from build123d import *

# Parameters (mm, degrees)
F0_R     = 63.5
F1_DEPTH = 7.62
F2_R     = 12.7
F3_DEPTH = 7.621


with BuildPart() as f1:
    # F0 (on Front) → F1 (new body)
    with BuildSketch(Plane.XZ):
        Circle(F0_R)
    extrude(amount=F1_DEPTH)

    # F2 (on Front) → F3 (cut, through all)
    with BuildSketch(Plane.XZ):
        with Locations((-28.595986, 36.92016)):
            Circle(F2_R)
        with Locations((-43.949804, -15.787442)):
            Circle(F2_R)
        with Locations((1.433513, -46.677336)):
            Circle(F2_R)
        with Locations((44.835764, -13.060738)):
            Circle(F2_R)
        with Locations((26.276513, 38.605356)):
            Circle(F2_R)
    extrude(amount=F3_DEPTH, mode=Mode.SUBTRACT)


solid = f1.part
Input: part model. Units: mm. Frame: model coordinates. Coordinates: 2 decimals unless noted, no trailing zeros. Loops run counter-clockwise (first coordinate to the right, second up) from the corner with the lowest first, then second, coordinate; pieces in that order, holes last. Notation, with made-up numbers: (41, 11) -> (79, 11) arc R24 cw to (79, 33) -> close; hole circle Ø9 at (40.5, 16.25). An arc over 180 degrees is marked (long way). Write item = value, one per line. Start each with the question number.
Item 1: Cut plane B-B, the plane z = 31. Return loops of the section in (x, y).
Item 2: First-contact query: P1, Ø1.5, axis at y = -4, z = 43.5, coming from the +X side; P2, Ø2, axis at y = -4.5, z = 39, coming from the +X side. Flat tips, straight axial feed; report the tip coordinate or a pass-through.
Item 3: Cut plane A-A, the plane x = 16. Return loops of the section in (y, z), plus the area to 3 significant figures.
Item 4: Cut plane C-C, the plane y = -3.5. Return loops of the section in (x, z), plus the area to 3 significant figures.
Item 5: Cut plane D-D, the plane x = 0. Return loops of the section in (y, z).
Item 6: Material intervals for line 1 (Z direction, x = -37, y = -3.25); line 2 (X direction, y = -5.75, z = -9); line 3 (X direction, y = -4.5, z = 42), sorted ascending.
Item 7: Mould query, pull axis Z, two halves, no side actions, for faces 1 (the face through (-38.09, -3.757, -27.055)), 2 (the face through (-1, 0, 1)), 3 (the face through (-13.77, -3.76, -61.99)). Classes: pulls with the +Z half, pulls with the -Z half, needs draft (parallel to the pull), parting line crosses it, or undercut.
Ans:
q1.outline = (-55.42, -7.62) -> (-39.83, -7.62) -> (-39.83, 0) -> (-55.42, 0) -> close; (-17.36, -7.62) -> (16.11, -7.62) -> (16.11, 0) -> (-17.36, 0) -> close; (36.45, -7.62) -> (55.42, -7.62) -> (55.42, 0) -> (36.45, 0) -> close
q2.P1 = 46.95
q2.P2 = 50.87
q3.outline = (-7.62, -61.45) -> (0, -61.45) -> (0, 31.14) -> (-7.62, 31.14) -> close; (-7.62, 46.07) -> (0, 46.07) -> (0, 61.45) -> (-7.62, 61.45) -> close
q3.area = 823 mm²
q4.outline = circle Ø127 at (0, 0); hole circle Ø25.4 at (-43.95, -15.79); hole circle Ø25.4 at (-28.6, 36.92); hole circle Ø25.4 at (1.43, -46.68); hole circle Ø25.4 at (26.28, 38.61); hole circle Ø25.4 at (44.84, -13.06)
q4.area = 10,100 mm²
q5.outline = (-7.62, -63.5) -> (0, -63.5) -> (0, -59.3) -> (-7.62, -59.3) -> close; (-7.62, -34.06) -> (0, -34.06) -> (0, 63.5) -> (-7.62, 63.5) -> close
q6.line_1 = -51.61 to -26.42, -5.16 to 27.4, 46.44 to 51.61
q6.line_2 = -62.86 to -54.68, -33.22 to 32.8, 56.87 to 62.86
q6.line_3 = -47.63 to -40.24, -16.96 to 14.04, 38.51 to 47.63
q7.face_1 = undercut
q7.face_2 = needs draft
q7.face_3 = parting line crosses it
